```python
from build123d import *

# Parameters (mm, degrees)
F1_DEPTH = 25.4
F2_DEPTH = 88.9
F3_DEPTH = 142.24


with BuildPart() as f1:
    # F0 (on Front) → F1 (new body)
    with BuildSketch(Plane.XZ):
        with BuildLine():
            Line((228.6, 254), (-381, 254))
            Line((-381, 254), (-381, -254))
            Line((-381, -254), (228.6, -254))
            Line((228.6, -254), (228.6, -47.4305862601))
            Line((228.6, -47.4305862601), (-190.3648431942, -100.7860047317))
            ThreePointArc((-190.3648431942, -100.7860047317), (-304.7999771648, -0.0681183971), (-190.5, 100.8031249516))
            Line((-190.5, 100.8031249516), (228.6, 48.0014880722))
            Line((228.6, 48.0014880722), (228.6, 254))
        make_face()
        with BuildLine():
            Line((309.5625, 37.8011718568), (228.6, 48.0014880722))
            Line((228.6, 48.0014880722), (228.6, -47.4305862601))
            Line((228.6, -47.4305862601), (302.4409560086, -38.0268972104))
            ThreePointArc((302.4409560086, -38.0268972104), (266.8669251864, 3.5625602015), (309.5625, 37.8011718568))
        make_face()
        with BuildLine():
            Line((228.6, -47.4305862601), (228.6, 48.0014880722))
            Line((228.6, 48.0014880722), (-190.5, 100.8031249516))
            ThreePointArc((-190.5, 100.8031249516), (-127, 67.202083301), (-101.6, 0))
            ThreePointArc((-101.6, 0), (-126.9549610418, -67.1509793991), (-190.3648431942, -100.7860047317))
            Line((-190.3648431942, -100.7860047317), (228.6, -47.4305862601))
        make_face()
        with BuildLine():
            ThreePointArc((342.9, 0), (333.375, 25.2007812379), (309.5625, 37.8011718568))
            ThreePointArc((309.5625, 37.8011718568), (266.8669251864, 3.5625602015), (302.4409560086, -38.0268972104))
            Line((302.4409560086, -38.0268972104), (316.6146676198, -36.2218667249))
            ThreePointArc((316.6146676198, -36.2218667249), (335.6362516879, -22.37712184), (342.9, 0))
        make_face()
        with BuildLine():
            Line((316.6146676198, -36.2218667249), (302.4409560086, -38.0268972104))
            ThreePointArc((302.4409560086, -38.0268972104), (309.6131838022, -37.7947517744), (316.6146676198, -36.2218667249))
        make_face()
        with BuildLine():
            ThreePointArc((-101.6, 0), (-127, 67.202083301), (-190.5, 100.8031249516))
            ThreePointArc((-190.5, 100.8031249516), (-304.7999771648, -0.0681183971), (-190.3648431942, -100.7860047317))
            ThreePointArc((-190.3648431942, -100.7860047317), (-126.9549610418, -67.1509793991), (-101.6, 0))
        make_face()
        with BuildLine():
            Line((228.6, -47.4305862601), (228.6, 48.0014880722))
            Line((228.6, 48.0014880722), (-190.5, 100.8031249516))
            ThreePointArc((-190.5, 100.8031249516), (-127, 67.202083301), (-101.6, 0))
            ThreePointArc((-101.6, 0), (-126.9549610418, -67.1509793991), (-190.3648431942, -100.7860047317))
            Line((-190.3648431942, -100.7860047317), (228.6, -47.4305862601))
        make_face()
        with BuildLine():
            Line((309.5625, 37.8011718568), (228.6, 48.0014880722))
            Line((228.6, 48.0014880722), (228.6, -47.4305862601))
            Line((228.6, -47.4305862601), (302.4409560086, -38.0268972104))
            ThreePointArc((302.4409560086, -38.0268972104), (266.8669251864, 3.5625602015), (309.5625, 37.8011718568))
        make_face()
        with BuildLine():
            ThreePointArc((342.9, 0), (333.375, 25.2007812379), (309.5625, 37.8011718568))
            ThreePointArc((309.5625, 37.8011718568), (266.8669251864, 3.5625602015), (302.4409560086, -38.0268972104))
            Line((302.4409560086, -38.0268972104), (316.6146676198, -36.2218667249))
            ThreePointArc((316.6146676198, -36.2218667249), (335.6362516879, -22.37712184), (342.9, 0))
        make_face()
    extrude(amount=F1_DEPTH)

    # F0 (on Front) → F2 (join)
    with BuildSketch(Plane.XZ):
        with BuildLine():
            ThreePointArc((342.9, 0), (333.375, 25.2007812379), (309.5625, 37.8011718568))
            ThreePointArc((309.5625, 37.8011718568), (266.8669251864, 3.5625602015), (302.4409560086, -38.0268972104))
            Line((302.4409560086, -38.0268972104), (316.6146676198, -36.2218667249))
            ThreePointArc((316.6146676198, -36.2218667249), (335.6362516879, -22.37712184), (342.9, 0))
        make_face()
        with BuildLine():
            ThreePointArc((-101.6, 0), (-127, 67.202083301), (-190.5, 100.8031249516))
            ThreePointArc((-190.5, 100.8031249516), (-304.7999771648, -0.0681183971), (-190.3648431942, -100.7860047317))
            ThreePointArc((-190.3648431942, -100.7860047317), (-126.9549610418, -67.1509793991), (-101.6, 0))
        make_face()
        with BuildLine():
            Line((228.6, -47.4305862601), (228.6, 48.0014880722))
            Line((228.6, 48.0014880722), (-190.5, 100.8031249516))
            ThreePointArc((-190.5, 100.8031249516), (-127, 67.202083301), (-101.6, 0))
            ThreePointArc((-101.6, 0), (-126.9549610418, -67.1509793991), (-190.3648431942, -100.7860047317))
            Line((-190.3648431942, -100.7860047317), (228.6, -47.4305862601))
        make_face()
        with BuildLine():
            Line((309.5625, 37.8011718568), (228.6, 48.0014880722))
            Line((228.6, 48.0014880722), (228.6, -47.4305862601))
            Line((228.6, -47.4305862601), (302.4409560086, -38.0268972104))
            ThreePointArc((302.4409560086, -38.0268972104), (266.8669251864, 3.5625602015), (309.5625, 37.8011718568))
        make_face()
    extrude(amount=F2_DEPTH)

    # F0 (on Front) → F3 (join)
    with BuildSketch(Plane.XZ):
        with BuildLine():
            ThreePointArc((342.9, 0), (333.375, 25.2007812379), (309.5625, 37.8011718568))
            ThreePointArc((309.5625, 37.8011718568), (266.8669251864, 3.5625602015), (302.4409560086, -38.0268972104))
            Line((302.4409560086, -38.0268972104), (316.6146676198, -36.2218667249))
            ThreePointArc((316.6146676198, -36.2218667249), (335.6362516879, -22.37712184), (342.9, 0))
        make_face()
        with BuildLine():
            ThreePointArc((-101.6, 0), (-127, 67.202083301), (-190.5, 100.8031249516))
            ThreePointArc((-190.5, 100.8031249516), (-304.7999771648, -0.0681183971), (-190.3648431942, -100.7860047317))
            ThreePointArc((-190.3648431942, -100.7860047317), (-126.9549610418, -67.1509793991), (-101.6, 0))
        make_face()
    extrude(amount=F3_DEPTH)


solid = f1.part
```
Here's how the part is built. I have some questions about the finished solid (model axes, mm). A direction names the side the tool comes from. Coordinates: 2 decimals unless noted, no trailing zeros. Order: outer loops, then holes, each group sorted by start corner. A loop starts at its lowest first (then second) coordinate and runs counter-clockwise, first axis right, second up. Notation, with made-up numbers: (3.25, 51) -> (20.25, 51) arc R7 cw to (20.25, 60) -> close; hole circle Ø4 at (71, -33). An arc over 180 degrees is marked (long way). Return JSON: item names as keys, results as strings.
1) I'm going to push flat-ended pins straight in: P1, Ø7.5, axis at y = -8.5, z = -115.5, coming from the +X side; P2, Ø6, axis at x = -229, y = -116, coming from the +Z side; P3, Ø1, axis at x = 28, z = 127, coming from the -Y side. Where does each tip first touch, or does it pass through?
Conclusion:
{"P1": "stops at x = 228.6", "P2": "stops at z = 99.01", "P3": "stops at y = -25.4"}
2) Thinking about a two-plate mould opening in X: for faces 4 (the flat face through (-381, -13, 4)), 5 (the flat face through (228.6, -13, -152)), 6 (the flat face through (-72, -13, 254)), 7 (the flat face through (56, -88.9, 1)), which applies, +X half, -X half, draft (parallel to the pull), parting line (faces both ways), or undercut?
Conclusion:
{"face 4": "-X half", "face 5": "+X half", "face 6": "draft", "face 7": "undercut"}
3) If we section it at B-B on z = 0: List the corners of the cut face in (x, y) for me, plus the area to 3 significant figures.
Conclusion:
{"outline": "(-381, -25.4) -> (-304.8, -25.4) -> (-304.8, -142.24) -> (-101.6, -142.24) -> (-101.6, -88.9) -> (266.7, -88.9) -> (266.7, -142.24) -> (342.9, -142.24) -> (342.9, 0) -> (-381, 0) -> close", "area": "74,400 mm²"}
4) If we section it at C-C on y = -103: List the corners of the cut face in (x, z) for me.
Conclusion:
{"outline": "circle Ø203.2 at (-203.2, 0); (302.44, -38.03) -> (316.61, -36.22) arc R38.1 ccw (long way) to start"}
5) On a 3-axis mill with a long thin cutter (end or side, diameter ignored), from which of +Z, -Z, +X, -X, +Y, -Y can I reach the whole of each face in a straight line? I mean faces 1 (the cylindrical face through (-304.37, -95.98, 9.32)), 2 (the flat face through (-80, -13, -254)), 3 (the flat face through (228.6, -13, 150)). Say none if no direction works.
Conclusion:
{"face 1": "-Y", "face 2": "-Z, +X, -X, +Y, -Y", "face 3": "+Z, +X, +Y, -Y"}
6) If we section it at A-A on x = -203.2: List the corners of the cut face in (y, z) for me.
Conclusion:
{"outline": "(-142.24, -101.6) -> (-25.4, -101.6) -> (-25.4, -254) -> (0, -254) -> (0, 254) -> (-25.4, 254) -> (-25.4, 101.6) -> (-142.24, 101.6) -> close"}
7) If we section it at D-D on y = -47.5: List the corners of the cut face in (x, z) for me, plus the area to 3 significant figures.
Conclusion:
{"outline": "(-190.5, 100.8) arc R101.6 ccw (long way) to (-190.36, -100.79) -> (316.61, -36.22) arc R38.1 ccw to (309.56, 37.8) -> close", "area": "89,800 mm²"}
8) If I drill on probe 1 along Y at (x, z) = (-224, -119.5); probe 2 along X at (y, z) = (-93, -27); probe 3 along X at (y, z) = (-111.5, 5.5), over which ranges is the centre line in solid material (lowest first)?
Conclusion:
{"probe 1": "y = -25.4 to 0", "probe 2": "x = -301.15 to -105.25, 277.92 to 331.68", "probe 3": "x = -304.65 to -101.75, 267.1 to 342.5"}
